Work out the finished part from the listing and answer in its coordinate system (mm). A direction names the side the tool comes from. Coordinates: 2 decimals unless noted, no trailing zeros. Loops run counter-clockwise (first coordinate to the right, second up) from the corner with the lowest first, then second, coordinate; pieces in that order, holes last. Notation, with made-up numbers: (50.5, 69.25) - (95.5, 69.25) arc R11 cw to (95.5, 85.25) - close; hole circle Ø6 at (34.5, 21). An arc over 180 degrees is marked (long way). Write each question's results on one line, items separated by ' | '. Start each with the question number.
1. Which of the six approach directions +Z, -Z, +X, -X, +Y, -Y give full straight-line access (tool end or side, diameter ignored) to faces 5 (the cylindrical face through (-3.765, 7.552, -13.649)), 6 (the flat face through (0, 3, -13.95)), 7 (the cylindrical face through (0.795, 0.301, 13.665)), 8 (the cylindrical face through (3.749, 7.552, 13.665)), 9 (the flat face through (17.7, 7, 0))?
2. Determine the mould class of faces 1 (the flat face through (0, 3, 13.95)), 2 (the cylindrical face through (21.299, 4.816, 13.665)), 3 (the cylindrical face through (10.985, 5.115, -13.649)), 4 (the flat face through (4.05, 7, 0)) for opening direction X: released by +X, released by -X, zero draft, split by the parting line, or undercut.
3. A cutting plane is placed at C-C on z = -6.25. Determine the outline of the cut face in (x, y).
4. Each of these flat-tipped pins is pushed along its axis until it touches: P1, Ø7, axis at x = 7.5, z = -1.5, coming from the +Y side; P2, Ø2, axis at x = -5.5, z = 5.5, coming from the +Y side; P3, Ø3, axis at x = 14.5, y = 8, coming from the +Z side (3 decimals). Where does it stop, or does it pass through?
5. Find the intervals of material crossed by line 1 along X through (y, z) = (9, 9); line 2 along Y through (x, z) = (-16.5, -12.5), in increasing order. Write a range as [from, to].
6. A cutting plane is placed at A-A on y = 8. Determine the outline of the cut face in (x, z), then the cut area to 3 significant figures.
7. A cutting plane is placed at B-B on x = 15.5. Determine the outline of the cut face in (y, z).
from build123d import *

# Parameters (mm, degrees)
SKETCH_1_W      = 43.2
SKETCH_1_H      = 27.9
EXTRUDE_1_DEPTH = 5.4
SKETCH_2_W      = 8.1
SKETCH_2_H      = 27.9
SKETCH_2_W_2    = 3.9
EXTRUDE_2_DEPTH = 4.1
FILLET_1_R      = 1


with BuildPart() as part:
    # Эскиз1 → Бобышка-Вытянуть1 (new body)
    with BuildSketch(Plane(origin=(0, 0, 0), x_dir=(1, 0, 0), z_dir=(0, 1, 0))):
        Rectangle(SKETCH_1_W, SKETCH_1_H)
    extrude(amount=EXTRUDE_1_DEPTH)

    # Эскиз2 → Бобышка-Вытянуть2 (add)
    with BuildSketch(Plane(origin=(0, 5.4, 0), x_dir=(1, 0, 0), z_dir=(0, 1, 0))):
        Rectangle(SKETCH_2_W, SKETCH_2_H)
        with Locations((-19.65, 0)):
            Rectangle(SKETCH_2_W_2, SKETCH_2_H)
        with Locations((19.65, 0)):
            Rectangle(SKETCH_2_W_2, SKETCH_2_H)
    extrude(amount=EXTRUDE_2_DEPTH)

    # Скругление1
    fillet_1_edges = [part.edges().sort_by_distance(p)[0] for p in [
        (-10.875, 5.4, -13.95),
        (10.875, 5.4, 13.95),
        (4.05, 7.45, 13.95),
        (4.05, 7.45, -13.95),
        (-4.05, 7.45, -13.95),
        (-4.05, 7.45, 13.95),
        (-10.875, 5.4, 13.95),
        (-17.7, 7.45, 13.95),
        (-17.7, 7.45, -13.95),
        (10.875, 5.4, -13.95),
        (17.7, 7.45, -13.95),
        (17.7, 7.45, 13.95),
        (0, 0, 13.95),
        (-21.6, 0, 0),
        (0, 0, -13.95),
        (21.6, 4.75, 13.95),
        (-21.6, 4.75, 13.95),
        (-21.6, 4.75, -13.95),
        (21.6, 4.75, -13.95),
    ]]
    fillet(fillet_1_edges, radius=FILLET_1_R)


solid = part.part
Values:
1) face 5: -Z, +Y | face 6: -Z, +X, -X, +Y, -Y | face 7: +Z, +X, -X, -Y | face 8: +Z, +Y | face 9: +Z, -Z, +Y
2) face 1: zero draft | face 2: released by +X | face 3: undercut | face 4: undercut
3) outline: (-21.6, 1) arc R1 ccw to (-20.6, 0) - (21.6, 0) - (21.6, 9.5) - (17.7, 9.5) - (17.7, 5.4) - (4.05, 5.4) - (4.05, 9.5) - (-4.05, 9.5) - (-4.05, 5.4) - (-17.7, 5.4) - (-17.7, 9.5) - (-21.6, 9.5) - close
4) P1: y = 9.5 | P2: y = 5.4 | P3: through
5) line 1: [-21.6, -17.7], [-4.05, 4.05], [17.7, 21.6] | line 2: [0, 5.4]
6) outline: (-21.6, -12.95) arc R1 ccw to (-20.6, -13.95) - (-18.7, -13.95) arc R1 ccw to (-17.7, -12.95) - (-17.7, 12.95) arc R1 ccw to (-18.7, 13.95) - (-20.6, 13.95) arc R1 ccw to (-21.6, 12.95) - close; (-4.05, -12.95) arc R1 ccw to (-3.05, -13.95) - (3.05, -13.95) arc R1 ccw to (4.05, -12.95) - (4.05, 12.95) arc R1 ccw to (3.05, 13.95) - (-3.05, 13.95) arc R1 ccw to (-4.05, 12.95) - close; (17.7, -12.95) arc R1 ccw to (18.7, -13.95) - (20.6, -13.95) arc R1 ccw to (21.6, -12.95) - (21.6, 12.95) arc R1 ccw to (20.6, 13.95) - (18.7, 13.95) arc R1 ccw to (17.7, 12.95) - close | area: 441 mm^2
7) outline: (0, -12.95) arc R1 ccw to (1, -13.95) - (4.4, -13.95) arc R1 ccw to (5.4, -12.95) - (5.4, 12.95) arc R1 ccw to (4.4, 13.95) - (1, 13.95) arc R1 ccw to (0, 12.95) - close
